Model file for the job. Use its own axes, mm. Face numbers are marked on the shaded views. A direction names the side the tool comes from. Give positions to 0.01 mm unless a question says otherwise; leave off trailing zeros. Write each loop counter-clockwise with the first axis right and the second up, starting at its lowest first coordinate (ties: lowest second). Pieces come first, ordered by that corner, then holes.
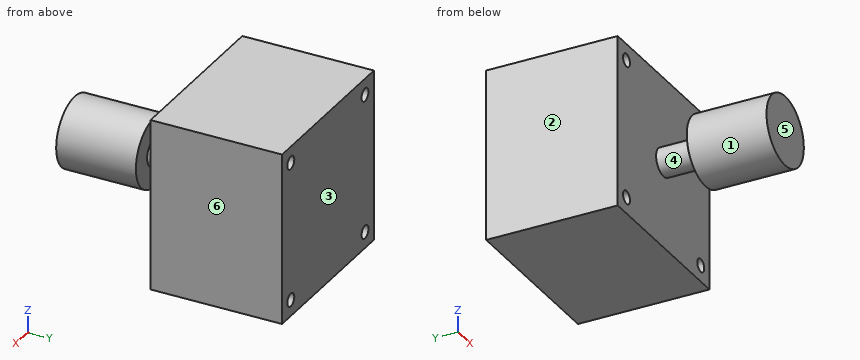
```python
from build123d import *

# Parameters (mm, degrees)
F0_W     = 86
F0_H     = 86
F0_R     = 3.25
F1_DEPTH = 66
F2_R     = 7
F3_DEPTH = 36
F5_R     = 17.5
F6_DEPTH = 40


with BuildPart() as f1:
    # F0 (on Front) → F1 (new body)
    with BuildSketch(Plane.XZ):
        Rectangle(F0_W, F0_H)
        with Locations((-34.75, -34.8)):
            Circle(F0_R, mode=Mode.SUBTRACT)
        with Locations((34.85, -34.8)):
            Circle(F0_R, mode=Mode.SUBTRACT)
        with Locations((-34.75, 34.8)):
            Circle(F0_R, mode=Mode.SUBTRACT)
        with Locations((34.85, 34.8)):
            Circle(F0_R, mode=Mode.SUBTRACT)
    extrude(amount=-F1_DEPTH)

    # F2 (on face) → F3 (join)
    with BuildSketch(Plane.XZ):
        Circle(F2_R)
    extrude(amount=F3_DEPTH)

    # F5 (on offset) → F6 (join)
    with BuildSketch(Plane(origin=(-0.000934, -21, 0), x_dir=(1, 0, 0), z_dir=(0, -1, 0))):
        Circle(F5_R)
    extrude(amount=F6_DEPTH)


solid = f1.part
```
1. Slice it at B-B, the plane z = -34.8. Write the cut outline in (x, y), and give its area (3 significant figures).
Calculated:
outline: (-43, 0) - (-38, 0) - (-38, 66) - (-43, 66) - close; (-31.5, 0) - (31.6, 0) - (31.6, 66) - (-31.5, 66) - close; (38.1, 0) - (43, 0) - (43, 66) - (38.1, 66) - close
area: 4,820 mm2
2. Slice it at D-D, the plane y = 36. Write the cut outline in (x, z).
Calculated:
outline: (-43, -43) - (43, -43) - (43, 43) - (-43, 43) - close; hole circle Ø6.5 at (-34.75, -34.8); hole circle Ø6.5 at (-34.75, 34.8); hole circle Ø6.5 at (34.85, -34.8); hole circle Ø6.5 at (34.85, 34.8)
3. Which spindle directions (+Z, -Z, +X, -X, +Y, -Y) get a long thin tool onto all of the face, cutting with end or side? Do the marked faces 1 and 2. Say none if no direction does.
Calculated:
face 1: -Y
face 2: +Z, -Z, -X, +Y, -Y
4. Probe probe 1 along X at (y, z) = (35, 35); probe 2 along Z at (x, y) = (34.85, 24.5); probe 3 along X at (y, z) = (51, -34). List the from-to ranges inside material, lowest first.
Calculated:
probe 1: x = -43 to -37.99, -31.51 to 31.61, 38.09 to 43
probe 2: z = -43 to -38.05, -31.55 to 31.55, 38.05 to 43
probe 3: x = -43 to -37.9, -31.6 to 31.7, 38 to 43
5. Pull direction Y, two halves, no side cores. Call the marked faces 3, 4, 5 and 6: +Y half, -Y half, draft (parallel to the pull), parting line (faces both ways), or undercut.
Calculated:
face 3: +Y half
face 4: undercut
face 5: -Y half
face 6: draft
6. Pin check, flat tips, straight feed: P1, Ø12, axis at y = -27.5, z = -1, coming from the -X side; P2, Ø2, axis at x = -27.5, z = -17.5, coming from the -Y side; P3, Ø3, axis at y = -39.5, z = 1, coming from the +X side. Stop position of each tip, or through.
Calculated:
P1: stops at x = -17.5
P2: stops at y = 0
P3: stops at x = 17.5
7. Slice it at C-C, the plane z = 0. Write the cut outline in (x, y).
Calculated:
outline: (-43, 0) - (-7, 0) - (-7, -21) - (-17.5, -21) - (-17.5, -61) - (17.5, -61) - (17.5, -21) - (7, -21) - (7, 0) - (43, 0) - (43, 66) - (-43, 66) - close
8. Slice it at A-A, the plane x = -34.75. Write the cut outline in (y, z), and give its area (3 significant figures).
Calculated:
outline: (0, -43) - (66, -43) - (66, -38.05) - (0, -38.05) - close; (0, -31.55) - (66, -31.55) - (66, 31.55) - (0, 31.55) - close; (0, 38.05) - (66, 38.05) - (66, 43) - (0, 43) - close
area: 4,820 mm2
